```python
from build123d import *

# Parameters (mm, degrees)
BOSS_EXTRUDE1_DEPTH     = 110
SKETCH2_W               = 30
SKETCH2_H               = 12.5
BOSS_EXTRUDE2_DEPTH     = 35
SKETCH3_R               = 8
CUT_EXTRUDE1_DEPTH      = 121.603742452
SKETCH4_R               = 1.5
SKETCH4_R_2             = 1.25
CUT_EXTRUDE2_DEPTH      = 12.5
SKETCH5_W               = 9.5
SKETCH5_H               = 12.5
CUT_EXTRUDE3_DEPTH      = 121.603742452
FILLET4_R               = 0.5
BOSS_EXTRUDE3_DEPTH     = 5
CUT_EXTRUDE4_DEPTH      = 158.919156753
CUT_EXTRUDE4_DEPTH_BACK = 158.919156753
SKETCH7_W               = 12
SKETCH7_H               = 12
SKETCH7_W_2             = 11
SKETCH7_H_2             = 22
SKETCH7_W_3             = 13.6
SKETCH7_H_3             = 7
BOSS_EXTRUDE4_START     = 5
BOSS_EXTRUDE4_DEPTH     = 5
CUT_EXTRUDE5_START      = -30
CUT_EXTRUDE5_DEPTH      = 30


# Read off the part's stored shape, not the designer's step: Cut-Extrude5
with BuildPart() as part:
    # Sketch1 → Boss-Extrude1 (new body)
    with BuildSketch(Plane.XY):
        with BuildLine():
            Line((13.568, -0.541666667), (18.568, -0.541666667))
            Line((18.568, -0.541666667), (18.568, 14.458333333))
            ThreePointArc((18.568, 14.458333333), (2.458872965, 53.349206299), (-36.432, 69.458333333))
            Line((-36.432, 69.458333333), (-69.432, 69.458333333))
            Line((-69.432, 69.458333333), (-69.432, 64.458333333))
            Line((-69.432, 64.458333333), (-36.432, 64.458333333))
            ThreePointArc((-36.432, 64.458333333), (-1.076660941, 49.813672393), (13.568, 14.458333333))
            Line((13.568, 14.458333333), (13.568, -0.541666667))
        make_face()
    extrude(amount=BOSS_EXTRUDE1_DEPTH)

    # Sketch2 → Boss-Extrude2 (add)
    with BuildSketch(Plane.ZY.offset(-13.568)):
        with Locations((55, 11.708333333)):
            Rectangle(SKETCH2_W, SKETCH2_H)
    extrude(amount=BOSS_EXTRUDE2_DEPTH)

    # Sketch3 → Cut-Extrude1 (cut, through all)
    with BuildSketch(Plane(origin=(0, 0, 40), x_dir=(-1, 0, 0), z_dir=(0, 0, -1))):
        with Locations((3.932, 5.458333333)):
            Circle(SKETCH3_R)
    extrude(amount=-CUT_EXTRUDE1_DEPTH, mode=Mode.SUBTRACT)

    # Sketch4 → Cut-Extrude2 (cut)
    with BuildSketch(Plane.XZ.offset(-5.458333333)):
        with Locations(Location((-17.932, 43.5, 0), (0, 0, 270))):
            Circle(SKETCH4_R)
        with Locations(Location((-17.932, 66.5, 0), (0, 0, 270))):
            Circle(SKETCH4_R)
        with Locations(Location((7.568, 43.5, 0), (0, 0, 270))):
            Circle(SKETCH4_R_2)
        with Locations(Location((7.568, 66.5, 0), (0, 0, 270))):
            Circle(SKETCH4_R_2)
    extrude(amount=-CUT_EXTRUDE2_DEPTH, mode=Mode.SUBTRACT)

    # Sketch5 → Cut-Extrude3 (cut, through all)
    with BuildSketch(Plane(origin=(0, 0, 40), x_dir=(-1, 0, 0), z_dir=(0, 0, -1))):
        with Locations((16.682, 11.708333333)):
            Rectangle(SKETCH5_W, SKETCH5_H)
    extrude(amount=-CUT_EXTRUDE3_DEPTH, mode=Mode.SUBTRACT)

    # Fillet4
    fillet4_edges = [part.edges().sort_by_distance(p)[0] for p in [
        (-11.932, 5.458333333, 55),
    ]]
    fillet(fillet4_edges, radius=FILLET4_R)

    # Sketch6 → Boss-Extrude3 (add)
    with BuildSketch(Plane.XY.offset(110)):
        with BuildLine():
            Line((18.332493433, 19.542648335), (-1.667506567, 19.542648335))
            Line((-1.667506567, 19.542648335), (-46.432, 29.458333333))
            Line((-46.432, 29.458333333), (-46.432, 39.458333333))
            Line((-46.432, 39.458333333), (-69.432, 39.458333333))
            Line((-69.432, 39.458333333), (-69.432, 69.458333333))
            Line((-69.432, 69.458333333), (-36.432, 69.458333333))
            ThreePointArc((-36.432, 69.458333333), (0.617714404, 55.1070561), (18.332493433, 19.542648335))
        make_face()
    extrude(amount=BOSS_EXTRUDE3_DEPTH)

    # Sketch7 → Cut-Extrude4 (cut, two sides: drawn at the far end of the back side and taken through both)
    with BuildSketch(Plane.ZY.offset(-13.568).offset(-CUT_EXTRUDE4_DEPTH_BACK)):
        with Locations((55, 23.958333333)):
            Rectangle(SKETCH7_W, SKETCH7_H)
        with Locations((95.5, 10.458333333)):
            Rectangle(SKETCH7_W_2, SKETCH7_H_2)
        with Locations((14.5, 10.458333333)):
            Rectangle(SKETCH7_W_2, SKETCH7_H_2)
        with Locations((79.8, 8.958333333)):
            Rectangle(SKETCH7_W_3, SKETCH7_H_3)
    extrude(amount=CUT_EXTRUDE4_DEPTH + CUT_EXTRUDE4_DEPTH_BACK, mode=Mode.SUBTRACT)

    # Sketch8 → Boss-Extrude4 (add)
    with BuildSketch(Plane(origin=(0, 0, 0), x_dir=(-1, 0, 0), z_dir=(0, 0, -1)).offset(BOSS_EXTRUDE4_START)):
        with BuildLine():
            Line((36.432, 69.458333333), (69.432, 69.458333333))
            Line((69.432, 69.458333333), (69.432, 64.458333333))
            Line((69.432, 64.458333333), (69.432, 39.458333333))
            Line((69.432, 39.458333333), (46.432, 39.458333333))
            Line((46.432, 39.458333333), (46.432, 29.458333333))
            Line((46.432, 29.458333333), (1.707690959, 19.958333333))
            Line((1.707690959, 19.958333333), (-18.292309041, 19.958333333))
            ThreePointArc((-18.292309041, 19.958333333), (-0.463121629, 55.247425012), (36.432, 69.458333333))
        make_face()
    extrude(amount=-BOSS_EXTRUDE4_DEPTH)

    # Cut-Extrude5 outline → Cut-Extrude5 (cut)
    with BuildSketch(Plane(origin=(0, 69.458333333, 0), x_dir=(1, 0, 0), z_dir=(0, 1, 0)).offset(CUT_EXTRUDE5_START)):
        Polygon((-23.932, -88.349364905), (-69.432, -9.541053161), (-69.432, -115), (-61.432, -115), (-61.432, -110), align=None)
    extrude(amount=CUT_EXTRUDE5_DEPTH, mode=Mode.SUBTRACT)


solid = part.part
```
Check sheet for the modelled part. Datum: model origin and axes. Units: mm. A direction names the side the tool comes from. Coordinates: 2 decimals unless noted, no trailing zeros. Loops run counter-clockwise (first coordinate to the right, second up) from the corner with the lowest first, then second, coordinate; pieces in that order, holes last. Notation, with made-up numbers: M 65,87.25 L 93,87.25 A26 ccw 93,117.25 Z; hole C -11.5,32.5 d11. An arc over 180 degrees is marked long. Answer as a JSON object with one key per item and string values.
1. Sectioned sample at C-C on y = 51.5. Record the cut outline in (x, z).
Outcome:
{"outline": "M -69.43,-5 L 4.22,-5 L 4.22,115 L -61.43,115 L -61.43,110 L -2.85,110 L -2.85,0 L -69.43,0 Z"}
2. Sectioned sample at B-B on z = 79. Record the cut outline in (x, y), and give its area (3 significant figures).
Outcome:
{"outline": "M -29.33,63.95 A50 cw 13.57,14.46 L 13.57,12.46 L 18.57,12.46 L 18.57,14.46 A55 ccw -29.33,69 Z; M 13.57,-0.54 L 18.57,-0.54 L 18.57,5.46 L 13.57,5.46 Z", "area": "417 mm²"}
3. Access from +Z, -Z, +X, -X, +Y, -Y to the whole of each face (thin tool, end or side, straight path). Record for faces 1 (the flat face through (-42.9, 66.9, 99.3)), 2 (the flat face through (16, 12.458, 80)), 3 (the flat face through (13.568, 5, 55)), 4 (the flat face through (8, 19.958, -3)).
Outcome:
{"face 1": "-X, +Y, -Y", "face 2": "+X, -X", "face 3": "-X, -Y", "face 4": "-Z, +X, -X, -Y"}
4. Scan lines: L1, parallel to Z at x = -33, y = 40.5; L2, parallel to X at y = 9.75, z = 66.5; L3, parallel to X at y = 16, z = 80. Record each from-to range of solid material in increasing order. Write a range as from..to.
Outcome:
{"L1": "-5..0, 110..115", "L2": "-11.93..-10.68, 2.82..6.32, 8.82..18.57", "L3": "13.54..18.55"}
5. Depth check by flat-ended pin: P1, Ø16.5, axis at y = 7, z = 53, coming from the -X side; P2, Ø3, axis at y = 27.5, z = 36.5, coming from the +X side; P3, Ø1.5, axis at x = 16.5, z = 16, coming from the -Y side. Enter the tip coordinate at first touch or a pass-through.
Outcome:
{"P1": "x = -11.93", "P2": "x = 17.34", "P3": "y = 21.46"}
6. Sectioned sample at D-D on z = 28.5. Record the cut outline in (x, y).
Outcome:
{"outline": "M -58.49,64.46 L -36.43,64.46 A50 cw 13.57,14.46 L 13.57,-0.54 L 18.57,-0.54 L 18.57,14.46 A55 ccw -36.43,69.46 L -58.49,69.46 Z"}
7. Sectioned sample at A-A on x = -50. Record the cut outline in (y, z).
Outcome:
{"outline": "M 39.46,-5 L 69.46,-5 L 69.46,43.2 L 64.46,43.2 L 64.46,0 L 39.46,0 Z; M 39.46,110 L 64.46,110 L 64.46,103.4 L 69.46,103.4 L 69.46,115 L 39.46,115 Z"}
8. Release check for a two-part mould opening along Z. For faces 5 (the flat face through (-29, 43, 0)), 6 (the flat face through (-26, 45, -5)), 7 (the flat face through (18.568, 7, 55)) record: pulls with the +Z half, pulls with the -Z half, needs draft (parallel to the pull), parting line crosses it, or undercut.
Outcome:
{"face 5": "undercut", "face 6": "pulls with the -Z half", "face 7": "needs draft"}
